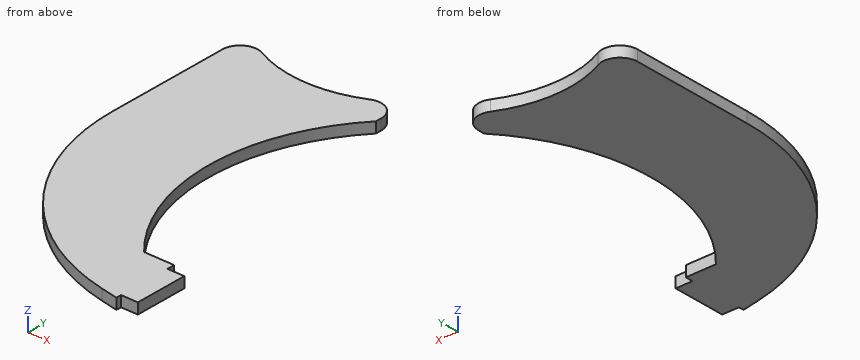
```python
from build123d import *

# Parameters (mm, degrees)
BOSS_EXTRUDE1_DEPTH = 6
FILLET1_R           = 10
FILLET2_R           = 10


with BuildPart() as part:
    # Sketch1 → Boss-Extrude1 (new body)
    with BuildSketch(Plane.XY):
        with BuildLine():
            Line((-79.123154231, -194.789726066), (-79.123154231, -164.789726066))
            Line((-79.123154231, -164.789726066), (-88.623154231, -164.789726066))
            Line((-88.623154231, -164.789726066), (-88.623154231, -160.48699252))
            Line((-88.623154231, -160.48699252), (-105.686834952, -160.48699252))
            ThreePointArc((-105.686834952, -160.48699252), (-134.328154399, -85.664912136), (-105.686834952, -10.842831751))
            Line((-105.686834952, -10.842831751), (-105.686834952, 11.052996518))
            ThreePointArc((-105.686834952, 11.052996518), (-150.657550595, -5.512129368), (-195.628266239, 11.052996518))
            Line((-195.628266239, 11.052996518), (-195.628266239, -78.076028691))
            ThreePointArc((-195.628266239, -78.076028691), (-168.199517459, -154.434154962), (-98.45220878, -195.885483519))
            Line((-98.45220878, -195.885483519), (-88.623154231, -197.789726066))
            Line((-88.623154231, -197.789726066), (-88.623154231, -194.789726066))
            Line((-88.623154231, -194.789726066), (-79.123154231, -194.789726066))
        make_face()
    extrude(amount=BOSS_EXTRUDE1_DEPTH)

    # Fillet1
    fillet1_edges = [part.edges().sort_by_distance(p)[0] for p in [
        (-195.628266239, 11.052996518, 3),
    ]]
    fillet(fillet1_edges, radius=FILLET1_R)

    # Fillet2
    fillet2_edges = [part.edges().sort_by_distance(p)[0] for p in [
        (-105.686834952, 11.052996518, 3),
    ]]
    fillet(fillet2_edges, radius=FILLET2_R)


solid = part.part
```
Input: part model. Units: mm. Frame: model coordinates. Coordinates: 2 decimals unless noted, no trailing zeros. Loops run counter-clockwise (first coordinate to the right, second up) from the corner with the lowest first, then second, coordinate; pieces in that order, holes last.
Q1. Section A-A, the plane z = 1.35. Return the cut outline in (x, y).
Results are:
outline: (-195.63, -78.08) arc R120 ccw to (-98.45, -195.89) - (-88.62, -197.79) - (-88.62, -194.79) - (-79.12, -194.79) - (-79.12, -164.79) - (-88.62, -164.79) - (-88.62, -160.49) - (-105.69, -160.49) arc R112.05 cw to (-105.69, -10.84) - (-105.69, -7.39) arc R10 ccw to (-120.1, 1.59) arc R69.33 cw to (-181.22, 1.59) arc R10 ccw to (-195.63, -7.39) - close
Q2. Section D-D, the plane x = -185. Return the cut outline in (y, z).
Results are:
outline: (-127.45, 0) - (2.59, 0) - (2.59, 6) - (-127.45, 6) - close
Q3. Section B-B, the plane x = -123. Return the cut outline in (y, z), and give its area (3 significant figures).
Results are:
outline: (-188.33, 0) - (-134.76, 0) - (-134.76, 6) - (-188.33, 6) - close; (-36.57, 0) - (0.24, 0) - (0.24, 6) - (-36.57, 6) - close
area: 542 mm2
Q4. Line query: line 1 along Y through (x, z) = (-120, 0.3); line 2 along Y through (x, z) = (-120.5, 3.45); line 3 along Y through (x, z) = (-135, 1.6). Output: solid intervals per line, ascending.
Results are:
line 1: y = -189.57 to -140.49, -30.84 to 1.63
line 2: y = -189.37 to -139.59, -31.74 to 1.39
line 3: y = -182.36 to -3.72
Q5. Contact query for flat-ended pins moving along their axis: pin 1 (0.9 mm diameter, centred on y = -196, z = 2.5, fed in from +X); pin 2 (3 mm diameter, centred on y = -93.5, z = 1, fed in from -X); pin 3 (1.7 mm diameter, centred on y = -8.5, z = 3.5, fed in from +X). Output: stop coordinate, or through.
Results are:
pin 1: stops at x = -88.62
pin 2: stops at x = -194.82
pin 3: stops at x = -105.69
Q6. Section C-C, the plane y = -139.5. Return the cut outline in (x, z), and give its area (3 significant figures).
Results are:
outline: (-178.72, 0) - (-120.55, 0) - (-120.55, 6) - (-178.72, 6) - close
area: 349 mm2
